Answer from the drawing. Dimensions are ordinates in mm from the lowest x, y and z of the part. A direction names the side the tool comes from. Coordinates: 2 decimals unless noted, no trailing zeros. Order: outer loops, then holes, each group sorted by start corner. A loop starts at its lowest first (then second) coordinate and runs counter-clockwise, first axis right, second up. Notation, with made-up numbers: (4, 39.5) - (60, 39.5) arc R19 ccw to (60, 63.5) - close; hole circle Ø8 at (-6.5, -18). An arc over 180 degrees is marked (long way). Answer as a JSON object with one key per item and string values. Group by question number.
1) Section B-B (x = 44.5) is taken. Give the vertices of the cut face in (y, z), plus the area to 3 significant figures.
2) The mould has two halves that part along Z. Classify the marked faces 1, 2 and 3: released by +Z, released by -Z, zero draft, split by the parting line, or undercut.
3) Each of these flat-tipped pins is pushed along its axis until it touches: P1, Ø1, axis at y = 9.5, z = 43.5, coming from the +X side; P2, Ø7, axis at y = 9.47, z = 78.21, coming from the -X side; P3, Ø3.5, axis at x = 55, z = 71, coming from the +Y side. Where does it stop, or does it pass through?
4) A tool of negligible diameter and unlimited length cuts with its end or side. For the marked faces 4, 5 and 6, from which of +Z, -Z, +X, -X, +Y, -Y can it reach the whole face along a straight path? Write none if from no direction.
5) Find the intervals of material crossed by line 1 along X through (y, z) = (10, 73.5); line 2 along Z through (x, y) = (47, 7.5) (1 decimal); line 3 along X through (y, z) = (8.5, 36.5), in increasing order.
6) Section D-D (z = 73.5) is taken. Give the vertices of the cut face in (x, y).
7) Section A-A (z = 12) is taken. Give the vertices of the cut face in (x, y) (1 decimal), plus the area to 3 significant figures.
8) Section C-C (y = 5.5) is taken. Give the vertices of the cut face in (x, z) (1 decimal).
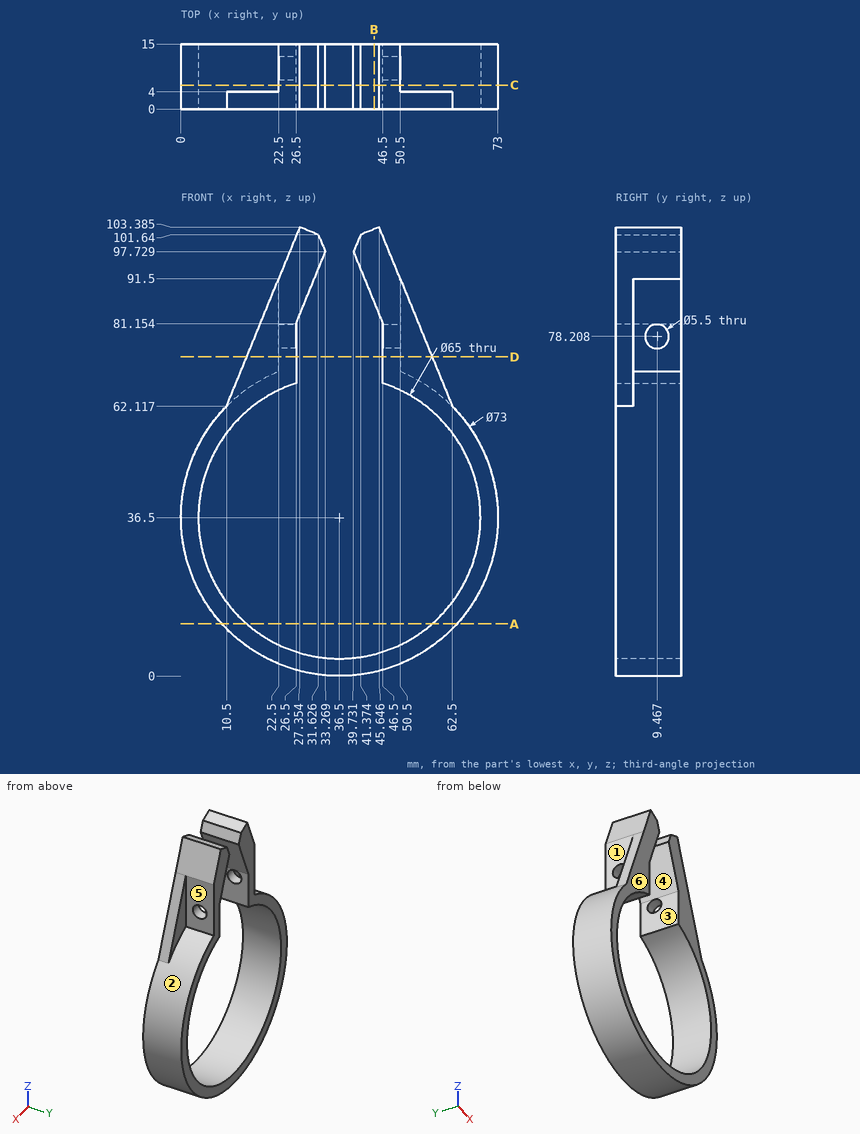
Report:
{
 "1": {"outline": "(0, 0.89) - (15, 0.89) - (15, 5) - (0, 5) - close; (0, 86.05) - (15, 86.05) - (15, 102.92) - (0, 102.92) - close", "area": "315 mm²"},
 "2": {"face 1": "zero draft", "face 2": "split by the parting line", "face 3": "undercut"},
 "3": {"P1": "stops at x = 72.42", "P2": "stops at x = 22.5", "P3": "stops at y = 4"},
 "4": {"face 4": "+Y, -Y", "face 5": "+Z, +X, +Y", "face 6": "+Z, -Z, +X, -X, -Y"},
 "5": {"line 1": "x = 22.5 to 26.5, 46.5 to 50.5", "line 2": "z = 1.5 to 5.7, 67.3 to 76.3, 80.1 to 100.1", "line 3": "x = 0 to 4, 69 to 73"},
 "6": {"outline": "(15.15, 0) - (26.5, 0) - (26.5, 15) - (22.5, 15) - (22.5, 4) - (15.15, 4) - close; (46.5, 0) - (57.85, 0) - (57.85, 4) - (50.5, 4) - (50.5, 15) - (46.5, 15) - close"},
 "7": {"outline": "(9.4, 0) - (15.1, 0) - (15.1, 15) - (9.4, 15) - close; (57.9, 0) - (63.6, 0) - (63.6, 15) - (57.9, 15) - close", "area": "171 mm²"},
 "8": {"outline": "(22.5, 70.2) arc R36.5 ccw (long way) to (50.5, 70.2) - (50.5, 91.5) - (45.6, 103.4) - (41.4, 101.6) - (39.7, 97.7) - (46.5, 81.2) - (46.5, 67.4) arc R32.5 cw (long way) to (26.5, 67.4) - (26.5, 81.2) - (33.3, 97.7) - (31.6, 101.6) - (27.4, 103.4) - (22.5, 91.5) - close"}
}
